Work out the finished part from the listing and answer in its coordinate system (mm). A direction names the side the tool comes from. Round coordinates to 2 decimals unless told otherwise and drop trailing zeros. Loops run counter-clockwise (first coordinate to the right, second up) from the corner with the lowest first, then second, coordinate; pieces in that order, holes last. Notation, with made-up numbers: M 67,77.25 L 100,77.25 A16 cw 100,81.25 Z; hole C 55,-39.5 d7. An arc over 180 degrees is marked long. One line per item, written item: value.
```python
from build123d import *

# Parameters (mm, degrees)
F0_W     = 50.8
F0_H     = 25.4
F1_DEPTH = 228.6
F2_R     = 2.5527
F3_DEPTH = 76.2
F4_W     = 47.6123
F4_H     = 22.2123
F5_DEPTH = 508
F6_R     = 2.5527
F7_DEPTH = 508


with BuildPart() as f1:
    # F0 (on Front) → F1 (new body)
    with BuildSketch(Plane.XZ):
        with Locations((2e-06, -54.285569)):
            Rectangle(F0_W, F0_H)
    extrude(amount=F1_DEPTH)

    # F2 (on face) → F3 (cut)
    with BuildSketch(Plane(origin=(0, 0, -66.985569), x_dir=(1, 0, 0), z_dir=(0, 0, -1))):
        with Locations((-12.699998, 215.9)):
            Circle(F2_R)
        with Locations((-12.699998, 190.5)):
            Circle(F2_R)
        with Locations((-12.699998, 165.1)):
            Circle(F2_R)
        with Locations((-12.699998, 139.7)):
            Circle(F2_R)
        with Locations((-12.699998, 114.3)):
            Circle(F2_R)
        with Locations((-12.699998, 88.9)):
            Circle(F2_R)
        with Locations((12.700002, 215.9)):
            Circle(F2_R)
        with Locations((12.700002, 190.5)):
            Circle(F2_R)
        with Locations((12.700002, 165.1)):
            Circle(F2_R)
        with Locations((12.700002, 139.7)):
            Circle(F2_R)
        with Locations((12.700002, 114.3)):
            Circle(F2_R)
        with Locations((12.700002, 88.9)):
            Circle(F2_R)
        with Locations((-12.699998, 63.5)):
            Circle(F2_R)
        with Locations((12.700002, 63.5)):
            Circle(F2_R)
        with Locations((-12.699998, 38.1)):
            Circle(F2_R)
        with Locations((12.700002, 38.1)):
            Circle(F2_R)
        with Locations((-12.699998, 12.7)):
            Circle(F2_R)
        with Locations((12.700002, 12.7)):
            Circle(F2_R)
    extrude(amount=-F3_DEPTH, mode=Mode.SUBTRACT)

    # F4 (on face) → F5 (cut)
    with BuildSketch(Plane.XZ.offset(228.6)):
        with Locations((0.006352, -54.291919)):
            Rectangle(F4_W, F4_H)
    extrude(amount=-F5_DEPTH, mode=Mode.SUBTRACT)

    # F6 (on face) → F7 (cut)
    with BuildSketch(Plane(origin=(-25.399998, 0, 0), x_dir=(0, -1, 0), z_dir=(-1, 0, 0))):
        with Locations((215.9, -54.285569)):
            Circle(F6_R)
        with Locations((190.5, -54.285569)):
            Circle(F6_R)
        with Locations((165.1, -54.285569)):
            Circle(F6_R)
        with Locations((139.7, -54.285569)):
            Circle(F6_R)
        with Locations((114.3, -54.285569)):
            Circle(F6_R)
        with Locations((88.9, -54.285569)):
            Circle(F6_R)
        with Locations((63.5, -54.285569)):
            Circle(F6_R)
        with Locations((38.1, -54.285569)):
            Circle(F6_R)
        with Locations((12.7, -54.285569)):
            Circle(F6_R)
    extrude(amount=-F7_DEPTH, mode=Mode.SUBTRACT)


solid = f1.part
```
1) Find section B-B (x = 21). Give the vertices of the cut face in (y, z).
Check values:
outline: M -228.6,-66.99 L 0,-66.99 L 0,-65.4 L -228.6,-65.4 Z; M -228.6,-43.19 L 0,-43.19 L 0,-41.59 L -228.6,-41.59 Z
2) The mould has two halves that part along Z. Classify faces 3 (the face through (-24.611, -40.535, -53.519)), 4 (the face through (-2, 0, -66)), 5 (the face through (0, -113, -66.986)): +Z half, -Z half, draft (parallel to the pull), parting line (faces both ways), or undercut.
Check values:
face 3: undercut
face 4: draft
face 5: -Z half
3) Find the intervals of material crossed by probe 1 along X at (y, z) = (-215.9, -42.2); probe 2 along X at (y, z) = (-156.5, -63); probe 3 along Z at (x, y) = (-13.5, -170.5), in increasing order. Write a range as from..to.
Check values:
probe 1: -25.4..-15.25, -10.15..10.15, 15.25..25.4
probe 2: -25.4..-23.8, 23.81..25.4
probe 3: -66.99..-65.4, -43.19..-41.59
4) Find section A-A (z = -63.5). Give the vertices of the cut face in (x, y), then the cut area to 3 significant figures.
Check values:
outline: M -25.4,-228.6 L -23.8,-228.6 L -23.8,0 L -25.4,0 Z; M 23.81,-228.6 L 25.4,-228.6 L 25.4,0 L 23.81,0 Z
area: 729 mm2
5) This flat-tipped pin is pushed along its axis until it touches: pin 1 (8 mm diameter, centred on x = -16, z = -57.5, fed in from +Y). Where does it stop, or does it pass through?
Check values:
pin 1: through
6) Find section D-D (y = -82). Give the vertices of the cut face in (x, z).
Check values:
outline: M -25.4,-66.99 L 25.4,-66.99 L 25.4,-41.59 L -25.4,-41.59 Z; hole M -23.8,-65.4 L 23.81,-65.4 L 23.81,-43.19 L -23.8,-43.19 Z
7) For faces 1 (the face through (0, -116, -43.186)), 2 (the face through (-13.253, -35.608, -66.203)), determine the directions among +Z, -Z, +X, -X, +Y, -Y from which every point of the face is accessible in a straight line to the end or side of a thin tool.
Check values:
face 1: +Y, -Y
face 2: +Z, -Z
8) Find section C-C (y = -38.1). Give the number of separate pieces and of enclosed holes in the cut face, then the cut area to 3 significant figures.
Check values:
separate pieces: 6
enclosed holes: 0
area: 184 mm2
